Verification items for the finished model (mm, model axes). A direction names the side the tool comes from. Coordinates: 2 decimals unless noted, no trailing zeros. Order: outer loops, then holes, each group sorted by start corner. A loop starts at its lowest first (then second) coordinate and runs counter-clockwise, first axis right, second up. Notation, with made-up numbers: (78, 22.25) -> (108, 22.25) arc R24 cw to (108, 44.25) -> close; hole circle Ø10 at (-1, -16.75). An arc over 180 degrees is marked (long way). Write item = value, one per line. Start each with the question number.
from build123d import *

# Parameters (mm, degrees)
F0_W      = 39.178138
F0_H      = 3.5
F0_W_2    = 40.821862
F1_DEPTH  = 5
F2_W      = 80
F2_H      = 4
F2_W_2    = 33.202673
F3_DEPTH  = 12
F4_W      = 7.437948
F4_H      = 4
F5_DEPTH  = 12
F6_W      = 38
F6_H      = 4
F7_DEPTH  = 12
F8_W      = 38
F8_H      = 4
F9_DEPTH  = 12
F10_W     = 38
F10_H     = 4
F11_DEPTH = 12
F12_W     = 38
F12_H     = 4
F13_DEPTH = 12
F14_W     = 38
F14_H     = 4
F15_DEPTH = 12
F16_W     = 38
F16_H     = 4
F17_DEPTH = 12
F18_W     = 38
F18_H     = 4
F19_DEPTH = 12
F20_W     = 80
F20_H     = 4
F21_DEPTH = 12
F22_W     = 38
F22_H     = 4
F23_DEPTH = 12
F24_W     = 38
F24_H     = 4
F25_DEPTH = 12
F26_W     = 38
F26_H     = 4
F27_DEPTH = 25
F28_W     = 38
F28_H     = 4
F29_DEPTH = 25


with BuildPart() as f1:
    # F0 (on Front) → F1 (new body)
    with BuildSketch(Plane.XZ):
        Polygon((0.805769, 45.985782), (-43.644231, 45.985782), (-43.644231, -55.614218), (0.805769, -55.614218), (0.805769, 37.953567), (-38.372369, 37.953567), (-38.372369, 41.453567), (0.805769, 41.453567), align=None)
        Polygon((45.255769, 45.985782), (0.805769, 45.985782), (0.805769, 41.453567), (41.627631, 41.453567), (41.627631, 37.953567), (0.805769, 37.953567), (0.805769, -55.614218), (45.255769, -55.614218), align=None)
        with Locations((-18.7833, 39.703567)):
            Rectangle(F0_W, F0_H)
        with Locations((21.2167, 39.703567)):
            Rectangle(F0_W_2, F0_H)
    extrude(amount=F1_DEPTH)

    # F2 (on face) → F3 (cut)
    with BuildSketch(Plane.XZ.offset(5)):
        with Locations((0.72034, 8.914189)):
            Rectangle(F2_W, F2_H)
        with Locations((1.153096, 24.914189)):
            Rectangle(F2_W, F2_H)
        with Locations((0.755769, -39.085811)):
            Rectangle(F2_W, F2_H)
        with Locations((0.805769, 40.914189)):
            Rectangle(F2_W, F2_H)
        with Locations((1.011494, -7.085811)):
            Rectangle(F2_W, F2_H)
        with Locations((-22.245567, 32.914189)):
            Rectangle(F2_W_2, F2_H)
    extrude(amount=-F3_DEPTH, mode=Mode.SUBTRACT)

    # F4 (on face) → F5 (cut)
    with BuildSketch(Plane.XZ.offset(5)):
        with Locations((-39.925257, 32.914189)):
            Rectangle(F4_W, F4_H)
    extrude(amount=-F5_DEPTH, mode=Mode.SUBTRACT)

    # F6 (on face) → F7 (cut)
    with BuildSketch(Plane.XZ.offset(5)):
        with Locations((26.255769, 32.914189)):
            Rectangle(F6_W, F6_H)
    extrude(amount=-F7_DEPTH, mode=Mode.SUBTRACT)

    # F8 (on face) → F9 (cut)
    with BuildSketch(Plane.XZ.offset(5)):
        with Locations((-24.644231, 16.914189)):
            Rectangle(F8_W, F8_H)
    extrude(amount=-F9_DEPTH, mode=Mode.SUBTRACT)

    # F10 (on face) → F11 (cut)
    with BuildSketch(Plane.XZ.offset(5)):
        with Locations((26.255769, 16.914189)):
            Rectangle(F10_W, F10_H)
    extrude(amount=-F11_DEPTH, mode=Mode.SUBTRACT)

    # F12 (on face) → F13 (cut)
    with BuildSketch(Plane.XZ.offset(5)):
        with Locations((-24.644231, 0.914189)):
            Rectangle(F12_W, F12_H)
    extrude(amount=-F13_DEPTH, mode=Mode.SUBTRACT)

    # F14 (on face) → F15 (cut)
    with BuildSketch(Plane(origin=(0, 0, 0), x_dir=(-1, 0, 0), z_dir=(0, 1, 0))):
        with Locations((-26.255769, 0.914189)):
            Rectangle(F14_W, F14_H)
    extrude(amount=-F15_DEPTH, mode=Mode.SUBTRACT)

    # F16 (on face) → F17 (cut)
    with BuildSketch(Plane(origin=(0, 0, 0), x_dir=(-1, 0, 0), z_dir=(0, 1, 0))):
        with Locations((-26.255769, -15.085811)):
            Rectangle(F16_W, F16_H)
    extrude(amount=-F17_DEPTH, mode=Mode.SUBTRACT)

    # F18 (on face) → F19 (cut)
    with BuildSketch(Plane(origin=(0, 0, 0), x_dir=(-1, 0, 0), z_dir=(0, 1, 0))):
        with Locations((24.644231, -15.085811)):
            Rectangle(F18_W, F18_H)
    extrude(amount=-F19_DEPTH, mode=Mode.SUBTRACT)

    # F20 (on face) → F21 (cut)
    with BuildSketch(Plane(origin=(0, 0, 0), x_dir=(-1, 0, 0), z_dir=(0, 1, 0))):
        with Locations((-0.855769, -24.760461)):
            Rectangle(F20_W, F20_H)
    extrude(amount=-F21_DEPTH, mode=Mode.SUBTRACT)

    # F22 (on face) → F23 (cut)
    with BuildSketch(Plane(origin=(0, 0, 0), x_dir=(-1, 0, 0), z_dir=(0, 1, 0))):
        with Locations((-26.255769, -32.760461)):
            Rectangle(F22_W, F22_H)
    extrude(amount=-F23_DEPTH, mode=Mode.SUBTRACT)

    # F24 (on face) → F25 (cut)
    with BuildSketch(Plane(origin=(0, 0, 0), x_dir=(-1, 0, 0), z_dir=(0, 1, 0))):
        with Locations((24.644231, -32.760461)):
            Rectangle(F24_W, F24_H)
    extrude(amount=-F25_DEPTH, mode=Mode.SUBTRACT)

    # F26 (on face) → F27 (cut)
    with BuildSketch(Plane.XZ.offset(5)):
        with Locations((-24.644231, -47.085811)):
            Rectangle(F26_W, F26_H)
    extrude(amount=-F27_DEPTH, mode=Mode.SUBTRACT)

    # F28 (on face) → F29 (cut)
    with BuildSketch(Plane.XZ.offset(5)):
        with Locations((26.255769, -47.085811)):
            Rectangle(F28_W, F28_H)
    extrude(amount=-F29_DEPTH, mode=Mode.SUBTRACT)


solid = f1.part
Item 1: Section check C-C (y = -4.2). State how many separate pieces and enclosed holes the cut face has, then the cut area to 3 significant figures.
Item 2: Mould release check, pull along X, two halves, no side actions. Record for faces 1 (the flat face through (-43.644, -2, -52)), 2 (the flat face through (0, -3, 10.914)), 3 (the flat face through (26, -3, -45.086)): pulls with the +X half, pulls with the -X half, needs draft (parallel to the pull), parting line crosses it, or undercut.
Item 3: Section check D-D (z = -15.5). Record the boundary of the cut face in (x, y), then the cut area to 3 significant figures.
Item 4: Section check B-B (x = -4.5). Record the boundary of the cut face in (y, z), then the cut area to 3 significant figures.
Item 5: Thickness scan on line 1 (X direction, y = -2.3, z = -40); line 2 (X direction, y = -0.4, z = -26); line 3 (X direction, y = -2.1, z = 1.5). Record the ranges inside material, lowest first.
Item 6: Section check A-A (z = 9.5). Record the boundary of the cut face in (x, y), then the cut area to 3 significant figures.
Item 7: Gauge pin test, flat ends, axial feed: P1, Ø1.2, axis at y = -3, z = 17.5, coming from the +X side; P2, Ø1.2, axis at y = -2.5, z = 16, coming from the -X side. Record the tip position at first contact, or that the pin passes through.
Item 8: Tool access check on faces 4 (the flat face through (-5.644, -3, -47)), 5 (the flat face through (0, 0, -4)), 6 (the flat face through (45.256, -2, 25)), 7 (the flat face through (-38.989, -3, -7)), 8 (the flat face through (27, -2, 2.914)). Record the directions out of +Z, -Z, +X, -X, +Y, -Y that give a thin tool (end or side, any length) a straight path to the whole face; none if there is none.
Filled sheet:
q1.separate_pieces = 1
q1.enclosed_holes = 6
q1.area = 5,290 mm^2
q2.face_1 = pulls with the -X half
q2.face_2 = undercut
q2.face_3 = needs draft
q3.outline = (-5.64, -5) -> (7.26, -5) -> (7.26, 0) -> (-5.64, 0) -> close
q3.area = 64.5 mm^2
q4.outline = (-5, -55.61) -> (0, -55.61) -> (0, -41.09) -> (-5, -41.09) -> close; (-5, -37.09) -> (0, -37.09) -> (0, -26.76) -> (-5, -26.76) -> close; (-5, -22.76) -> (0, -22.76) -> (0, -9.09) -> (-5, -9.09) -> close; (-5, -5.09) -> (0, -5.09) -> (0, 6.91) -> (-5, 6.91) -> close; (-5, 10.91) -> (0, 10.91) -> (0, 22.91) -> (-5, 22.91) -> close; (-5, 26.91) -> (0, 26.91) -> (0, 38.91) -> (-5, 38.91) -> close; (-5, 42.91) -> (0, 42.91) -> (0, 45.99) -> (-5, 45.99) -> close
q4.area = 388 mm^2
q5.line_1 = -43.64 to -39.24, 40.76 to 45.26
q5.line_2 = -43.64 to -39.14, 40.86 to 45.26
q5.line_3 = -5.64 to 7.26
q6.outline = (-43.64, -5) -> (-39.28, -5) -> (-39.28, 0) -> (-43.64, 0) -> close; (40.72, -5) -> (45.26, -5) -> (45.26, 0) -> (40.72, 0) -> close
q6.area = 44.5 mm^2
q7.P1 = 7.26
q7.P2 = -5.64
q8.face_4 = -X, +Y, -Y
q8.face_5 = +Z, -Z, +X, -X, +Y
q8.face_6 = +Z, -Z, +X, +Y, -Y
q8.face_7 = +Y, -Y
q8.face_8 = +X, +Y, -Y
